from build123d import *

# Parameters (mm, degrees)
SKETCH1_W           = 65
SKETCH1_H           = 30
BOSS_EXTRUDE1_DEPTH = 5
SKETCH2_W           = 20
SKETCH2_H           = 15
BOSS_EXTRUDE2_DEPTH = 15
CUT_EXTRUDE1_DEPTH  = 15
SKETCH4_R           = 1.852641707
CUT_EXTRUDE2_DEPTH  = 39.810436741
SKETCH5_W           = 10
SKETCH5_H           = 30
BOSS_EXTRUDE3_DEPTH = 34.146213


with BuildPart() as part:
    # Sketch1 → Boss-Extrude1 (new body)
    with BuildSketch(Plane(origin=(0, 0, 0), x_dir=(1, 0, 0), z_dir=(0, 1, 0))):
        Rectangle(SKETCH1_W, SKETCH1_H)
    extrude(amount=BOSS_EXTRUDE1_DEPTH)

    # Sketch2 → Boss-Extrude2 (add)
    with BuildSketch(Plane(origin=(0, 5, 0), x_dir=(1, 0, 0), z_dir=(0, 1, 0))):
        with Locations((0, 7.5)):
            Rectangle(SKETCH2_W, SKETCH2_H)
    extrude(amount=BOSS_EXTRUDE2_DEPTH)

    # Sketch3 → Cut-Extrude1 (cut)
    with BuildSketch(Plane(origin=(0, 20, 0), x_dir=(1, 0, 0), z_dir=(0, 1, 0))):
        with BuildLine():
            Line((-5, 2.5), (5, 2.5))
            ThreePointArc((5, 2.5), (7.375699039, 7.5), (5, 12.5))
            Line((5, 12.5), (-5, 12.5))
            ThreePointArc((-5, 12.5), (-7.375699039, 7.5), (-5, 2.5))
        make_face()
    extrude(amount=-CUT_EXTRUDE1_DEPTH, mode=Mode.SUBTRACT)

    # Sketch4 → Cut-Extrude2 (cut, through all)
    with BuildSketch(Plane(origin=(0, 5, 0), x_dir=(1, 0, 0), z_dir=(0, 1, 0))):
        with Locations(Location((0, 7.5, 0), (0, 0, 270))):
            Circle(SKETCH4_R)
    extrude(amount=-CUT_EXTRUDE2_DEPTH, mode=Mode.SUBTRACT)

    # Sketch5 → Boss-Extrude3 (add)
    with BuildSketch(Plane.XZ):
        with Locations((27.5, 0)):
            Rectangle(SKETCH5_W, SKETCH5_H)
        with Locations((-27.5, 0)):
            Rectangle(SKETCH5_W, SKETCH5_H)
    extrude(amount=BOSS_EXTRUDE3_DEPTH)


solid = part.part
Could you check a few things on this model? Use its own coordinates, in mm. A direction names the side the tool comes from. Round coordinates to 2 decimals unless told otherwise and drop trailing zeros. Order: outer loops, then holes, each group sorted by start corner. A loop starts at its lowest first (then second) coordinate and runs counter-clockwise, first axis right, second up.
Q1. Thinking about a two-plate mould opening in Z: for faces 6 (the face through (32.5, -14, 0)), 7 (the face through (-5, 1, 15)), 8 (the face through (0, 13, -2.5)), which applies, released by +Z, released by -Z, zero draft, split by the parting line, or undercut?
Geometry says:
face 6: zero draft
face 7: released by +Z
face 8: undercut
Q2. Which directions (+Z, -Z, +X, -X, +Y, -Y) give clear straight access to the entire face, cutting with the end or side of a thin tool? Please do faces 1 (the face through (10, 12, -7)), 2 (the face through (-10, 12, -7)), 3 (the face through (0, 12, 0)), 4 (the face through (7.375, 12.605, -7.42)), 5 (the face through (22.5, -17, 0)).
Geometry says:
face 1: +Z, -Z, +X, +Y
face 2: +Z, -Z, -X, +Y
face 3: +Z, +X, -X, +Y
face 4: +Y
face 5: +Z, -Z, -Y
Q3. I'm going to push flat-ended pins straight in: P1, Ø12, axis at x = -15, y = -18, coming from the -Z side; P2, Ø4.5, axis at x = -1, y = 16, coming from the +Z side; P3, Ø8, axis at x = -16, z = -10.5, coming from the +Y side; P4, Ø2, axis at x = -10.5, z = 7.5, coming from the -Y side. Where does each tip first touch, or does it pass through?
Geometry says:
P1: passes through
P2: stops at z = 0
P3: stops at y = 5
P4: stops at y = 0
Q4. Imagine slicing it at D-D, the plane z = 9.75. List the corners of the cut face in (x, y) for me.
Geometry says:
outline: (-32.5, -34.15) - (-22.5, -34.15) - (-22.5, 0) - (22.5, 0) - (22.5, -34.15) - (32.5, -34.15) - (32.5, 5) - (-32.5, 5) - close
Q5. Imagine slicing it at A-A, the plane z = -7.5. List the corners of the cut face in (x, y) for me.
Geometry says:
outline: (-32.5, -34.15) - (-22.5, -34.15) - (-22.5, 0) - (-1.85, 0) - (-1.85, 5) - (-7.38, 5) - (-7.38, 20) - (-10, 20) - (-10, 5) - (-32.5, 5) - close; (1.85, 0) - (22.5, 0) - (22.5, -34.15) - (32.5, -34.15) - (32.5, 5) - (10, 5) - (10, 20) - (7.38, 20) - (7.38, 5) - (1.85, 5) - close
Q6. Please list where these lines run through material, in increasing order: probe 1 along X at (y, z) = (-16.5, -12.75); probe 2 along X at (y, z) = (1.1, -7.5); probe 3 along Y at (x, z) = (1, -2).
Geometry says:
probe 1: x = -32.5 to -22.5, 22.5 to 32.5
probe 2: x = -32.5 to -1.85, 1.85 to 32.5
probe 3: y = 0 to 20
Q7. Imagine slicing it at C-C, the plane x = 0. List the corners of the cut face in (y, z) for me, then the cut area to 3 significant figures.
Geometry says:
outline: (0, -15) - (20, -15) - (20, -12.5) - (5, -12.5) - (5, -9.35) - (0, -9.35) - close; (0, -5.65) - (5, -5.65) - (5, -2.5) - (20, -2.5) - (20, 0) - (5, 0) - (5, 15) - (0, 15) - close
area: 206 mm2
Q8. Imagine slicing it at B-B, the plane y = -4. List the corners of the cut face in (x, z) for me, then the cut area to 3 significant figures.
Geometry says:
outline: (-32.5, -15) - (-22.5, -15) - (-22.5, 15) - (-32.5, 15) - close; (22.5, -15) - (32.5, -15) - (32.5, 15) - (22.5, 15) - close
area: 600 mm2
